```python
from build123d import *

# Parameters (mm, degrees)
SKETCH7_R          = 6.985
CUT_EXTRUDE4_DEPTH = 12.7


with BuildPart() as part:
    # Sweep1: sweep along a path in Sketch2
    with BuildLine(Plane(origin=(0, 0, 0), x_dir=(1, 0, 0), z_dir=(0, 1, 0))) as sweep1_path:
        Line((0, 0), (0, -152.4))
    # Sketch1 → Sweep1 (sweep)
    with BuildSketch(Plane.XY):
        Polygon((0, 0), (0, 76.2), (12.7, 76.2), (12.7, 12.7), (152.4, 12.7), (152.4, 0), align=None)
    sweep(path=sweep1_path.line)

    # Sketch7 → Cut-Extrude4 (cut)
    with BuildSketch(Plane(origin=(12.7, 0, 0), x_dir=(0, 0, -1), z_dir=(1, 0, 0))):
        with Locations((-133.35, 28.575)):
            Circle(SKETCH7_R)
        with Locations((-19.05, 28.575)):
            Circle(SKETCH7_R)
        with Locations((-76.2, 60.325)):
            Circle(SKETCH7_R)
        with Locations((-76.2, 28.575)):
            Circle(SKETCH7_R)
    extrude(amount=-CUT_EXTRUDE4_DEPTH, mode=Mode.SUBTRACT)


solid = part.part
```
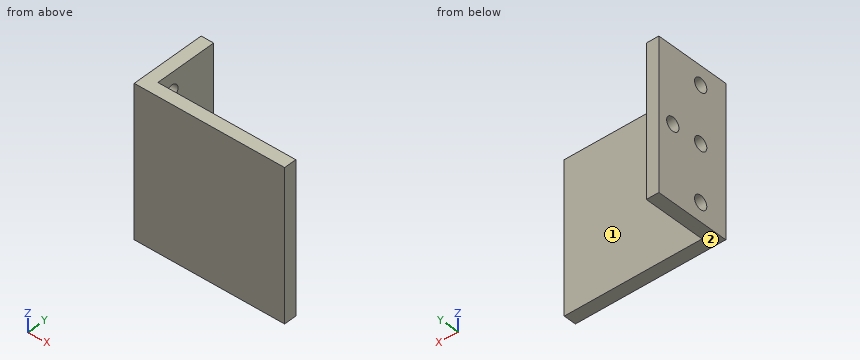
Build history of the part. All positions in model axes, mm. Face numbers are marked on the shaded views. A direction names the side the tool comes from. Give positions to 0.01 mm unless a question says otherwise; leave off trailing zeros. Loops run counter-clockwise (first coordinate to the right, second up) from the corner with the lowest first, then second, coordinate; pieces in that order, holes last. Notation, with made-up numbers: (-14, 5.25) - (43, 5.25) arc R19 ccw to (43, 21.25) - close; hole circle Ø6 at (27.5, 38). An arc over 180 degrees is marked (long way). Use a Markdown table: item, result.
(1) Band-saw the part on C-C (y = 18). Give the cut face in (x, z).
Taken from the geometry:
| item | result |
|---|---|
| outline | (0, 0) - (12.7, 0) - (12.7, 152.4) - (0, 152.4) - close |
(2) Wall check: line 1 along Y through (x, z) = (3, 19.05); line 2 along Y through (x, z) = (5.75, 76.2); line 3 along X through (y, z) = (58, 35.5). Give the ranges that are in metal, low to high.
Taken from the geometry:
| item | result |
|---|---|
| line 1 | 0 to 21.59, 35.56 to 76.2 |
| line 2 | 0 to 21.59, 35.56 to 53.34, 67.31 to 76.2 |
| line 3 | 0 to 12.7 |
(3) Which spindle directions (+Z, -Z, +X, -X, +Y, -Y) get a long thin tool onto all of the face, cutting with end or side? Do the marked faces 1 and 2. Say none if no direction does.
Taken from the geometry:
| item | result |
|---|---|
| face 1 | +Z, -Z, +X, +Y |
| face 2 | -Z, +X, -X, +Y, -Y |
(4) Band-saw the part on A-A (z = 133.35). Give the cut face in (x, y), and give its area (3 significant figures).
Taken from the geometry:
| item | result |
|---|---|
| outline | (0, 0) - (152.4, 0) - (152.4, 12.7) - (12.7, 12.7) - (12.7, 21.59) - (0, 21.59) - close; (0, 35.56) - (12.7, 35.56) - (12.7, 76.2) - (0, 76.2) - close |
| area | 2,560 mm2 |
(5) Band-saw the part on B-B (z = 76.2). Give the cut face in (x, y), and give its area (3 significant figures).
Taken from the geometry:
| item | result |
|---|---|
| outline | (0, 0) - (152.4, 0) - (152.4, 12.7) - (12.7, 12.7) - (12.7, 21.59) - (0, 21.59) - close; (0, 35.56) - (12.7, 35.56) - (12.7, 53.34) - (0, 53.34) - close; (0, 67.31) - (12.7, 67.31) - (12.7, 76.2) - (0, 76.2) - close |
| area | 2,390 mm2 |
(6) Drop flat-ended pins along their axis: pin 1 Ø19 at (y, z) = (39.5, 45) entering from +X; pin 2 Ø12.5 at (y, z) = (60.325, 76.2) entering from -X. Give the stop position or say it passes through.
Taken from the geometry:
| item | result |
|---|---|
| pin 1 | x = 12.7 |
| pin 2 | through |
